Model file for the job. Use its own axes, mm. A direction names the side the tool comes from. Give positions to 0.01 mm unless a question says otherwise; leave off trailing zeros. Loops run counter-clockwise (first coordinate to the right, second up) from the corner with the lowest first, then second, coordinate; pieces in that order, holes last. Notation, with made-up numbers: M 5,12.5 L 29,12.5 A25 cw 29,30.5 Z; hole C -22.5,69 d5. An arc over 180 degrees is marked long. Answer in a Markdown table with one row per item.
```python
from build123d import *

# Parameters (mm, degrees)
ESBO_O1_W                = 20
ESBO_O1_H                = 25
RESSALTO_EXTRUS_O1_DEPTH = 9
ESBO_O2_R                = 7.5
CORTE_EXTRUS_O1_DEPTH    = 29.390139133
FILETE1_R                = 3
RESSALTO_EXTRUS_O2_DEPTH = 6
RESSALTO_EXTRUS_O3_DEPTH = 6
FILETE3_R                = 1
FILETE5_R                = 3
FILETE6_R                = 1
ESBO_O5_W                = 4
ESBO_O5_H                = 6
RESSALTO_EXTRUS_O4_DEPTH = 8


with BuildPart() as part:
    # Esboço1 → Ressalto-extrusão1 (new body)
    with BuildSketch(Plane(origin=(0, 0, 0), x_dir=(1, 0, 0), z_dir=(0, 1, 0))):
        Rectangle(ESBO_O1_W, ESBO_O1_H)
    extrude(amount=RESSALTO_EXTRUS_O1_DEPTH)

    # Esboço2 → Corte-extrusão1 (cut, through all)
    with BuildSketch(Plane.XY.offset(12.5)):
        with Locations((0, 10)):
            Circle(ESBO_O2_R)
    extrude(amount=-CORTE_EXTRUS_O1_DEPTH, mode=Mode.SUBTRACT)

    # Filete1
    filete1_edges = [part.edges().sort_by_distance(p)[0] for p in [
        (-10, 0, 0),
        (10, 0, 0),
    ]]
    fillet(filete1_edges, radius=FILETE1_R)

    # Esboço3 → Ressalto-extrusão2 (add)
    with BuildSketch(Plane(origin=(0, 9, 0), x_dir=(1, 0, 0), z_dir=(0, 1, 0))):
        Polygon((-16, 10), (-10, 10), (-10, 8.5), (-14, 8.5), (-14, 6.5), (-10, 6.5), (-10, 5), (-16, 5), align=None)
        Polygon((-14, -6.5), (-10, -6.5), (-10, -5), (-16, -5), (-16, -10), (-10, -10), (-10, -8.5), (-14, -8.5), align=None)
    extrude(amount=-RESSALTO_EXTRUS_O2_DEPTH)

    # Esboço4 → Ressalto-extrusão3 (add)
    with BuildSketch(Plane(origin=(0, 9, 0), x_dir=(1, 0, 0), z_dir=(0, 1, 0))):
        Polygon((-16, -10), (-16, -5), (-11, -5), (-11, -6.5), (-14, -6.5), (-14, -8.5), (-11, -8.5), (-11, -10), align=None)
        Polygon((-11, 10), (-16, 10), (-16, 5), (-11, 5), (-11, 6.5), (-14, 6.5), (-14, 8.5), (-11, 8.5), align=None)
    extrude(amount=RESSALTO_EXTRUS_O3_DEPTH)

    # Filete3
    filete3_edges = [part.edges().sort_by_distance(p)[0] for p in [
        (-16, 9, -5),
        (-16, 9, -10),
        (-16, 9, 10),
        (-16, 9, 5),
    ]]
    fillet(filete3_edges, radius=FILETE3_R)

    # Filete5
    # the kernel refuses this fillet: 3 mm, written as the material it adds along each edge
    with BuildSketch(Plane(origin=(-10, 16.5, -5), x_dir=(-1, 0, 0), z_dir=(0, -1, 0))) as filete5_piece_1_section:
        with BuildLine():
            CenterArc((FILETE5_R, -FILETE5_R), FILETE5_R, 90, 90)
            Line((0, -FILETE5_R), (0, 0))
            Line((0, 0), (FILETE5_R, 0))
        make_face()
    filete5_piece_1 = extrude(amount=13.5, mode=Mode.PRIVATE)
    filete5_piece_1 = split(filete5_piece_1, bisect_by=Plane(origin=(-11.589070595, 9, -4.827479681), z_dir=(0, 1, 0)), keep=Keep.TOP, mode=Mode.PRIVATE)
    filete5_piece_1 = split(filete5_piece_1, bisect_by=Plane(origin=(-11, 12, -4.827479681), z_dir=(-1, 0, 0)), keep=Keep.TOP, mode=Mode.PRIVATE)
    filete5_piece_1 = split(filete5_piece_1, bisect_by=Plane(origin=(-11.589070595, 15, -4.827479681), z_dir=(0, -1, 0)), keep=Keep.TOP, mode=Mode.PRIVATE)
    add(filete5_piece_1)
    with BuildSketch(Plane(origin=(-10, 9, -5), x_dir=(-1, 0, 0), z_dir=(0, -1, 0))) as filete5_piece_2_section:
        with BuildLine():
            CenterArc((FILETE5_R, -FILETE5_R), FILETE5_R, 90, 90)
            Line((0, -FILETE5_R), (0, 0))
            Line((0, 0), (FILETE5_R, 0))
        make_face()
    filete5_piece_2 = extrude(amount=6, mode=Mode.PRIVATE)
    filete5_piece_2 = split(filete5_piece_2, bisect_by=Plane(origin=(-11, 6, -4.827479681), z_dir=(-1, 0, 0)), keep=Keep.TOP, mode=Mode.PRIVATE)
    add(filete5_piece_2)
    with BuildSketch(Plane(origin=(-10, 9, -5), x_dir=(-1, 0, 0), z_dir=(0, -1, 0))) as filete5_piece_3_section:
        with BuildLine():
            CenterArc((FILETE5_R, -FILETE5_R), FILETE5_R, 90, 90)
            Line((0, -FILETE5_R), (0, 0))
            Line((0, 0), (FILETE5_R, 0))
        make_face()
    filete5_piece_3 = extrude(amount=6, mode=Mode.PRIVATE)
    filete5_piece_3 = split(filete5_piece_3, bisect_by=Plane(origin=(-11, 6, -4.141402177), z_dir=(1, 0, 0)), keep=Keep.TOP, mode=Mode.PRIVATE)
    add(filete5_piece_3)
    with BuildSketch(Plane(origin=(-10, 16.5, 5), x_dir=(-1, 0, 0), z_dir=(0, -1, 0))) as filete5_piece_4_section:
        with BuildLine():
            CenterArc((FILETE5_R, FILETE5_R), FILETE5_R, 180, 90)
            Line((0, FILETE5_R), (0, 0))
            Line((0, 0), (FILETE5_R, 0))
        make_face()
    filete5_piece_4 = extrude(amount=13.5, mode=Mode.PRIVATE)
    filete5_piece_4 = split(filete5_piece_4, bisect_by=Plane(origin=(-11.589070595, 15, 4.827479681), z_dir=(0, -1, 0)), keep=Keep.TOP, mode=Mode.PRIVATE)
    filete5_piece_4 = split(filete5_piece_4, bisect_by=Plane(origin=(-11.589070595, 9, 4.827479681), z_dir=(0, 1, 0)), keep=Keep.TOP, mode=Mode.PRIVATE)
    filete5_piece_4 = split(filete5_piece_4, bisect_by=Plane(origin=(-11, 12, 4.827479681), z_dir=(-1, 0, 0)), keep=Keep.TOP, mode=Mode.PRIVATE)
    add(filete5_piece_4)
    with BuildSketch(Plane(origin=(-10, 9, 5), x_dir=(-1, 0, 0), z_dir=(0, -1, 0))) as filete5_piece_5_section:
        with BuildLine():
            CenterArc((FILETE5_R, FILETE5_R), FILETE5_R, 180, 90)
            Line((0, FILETE5_R), (0, 0))
            Line((0, 0), (FILETE5_R, 0))
        make_face()
    filete5_piece_5 = extrude(amount=6, mode=Mode.PRIVATE)
    filete5_piece_5 = split(filete5_piece_5, bisect_by=Plane(origin=(-11, 6, 4.827479681), z_dir=(-1, 0, 0)), keep=Keep.TOP, mode=Mode.PRIVATE)
    add(filete5_piece_5)
    with BuildSketch(Plane(origin=(-10, 9, 5), x_dir=(-1, 0, 0), z_dir=(0, -1, 0))) as filete5_piece_6_section:
        with BuildLine():
            CenterArc((FILETE5_R, FILETE5_R), FILETE5_R, 180, 90)
            Line((0, FILETE5_R), (0, 0))
            Line((0, 0), (FILETE5_R, 0))
        make_face()
    filete5_piece_6 = extrude(amount=6, mode=Mode.PRIVATE)
    filete5_piece_6 = split(filete5_piece_6, bisect_by=Plane(origin=(-11, 6, 4.141402177), z_dir=(1, 0, 0)), keep=Keep.TOP, mode=Mode.PRIVATE)
    add(filete5_piece_6)

    # Filete6
    filete6_edges = [part.edges().sort_by_distance(p)[0] for p in [
        (-11, 12, -4.236067977),
        (-11, 12, 4.236067977),
    ]]
    fillet(filete6_edges, radius=FILETE6_R)

    # Esboço5 → Ressalto-extrusão4 (add)
    with BuildSketch(Plane(origin=(10, 0, 0), x_dir=(0, 0, -1), z_dir=(1, 0, 0))):
        with Locations((-10.5, 6)):
            Rectangle(ESBO_O5_W, ESBO_O5_H)
    extrude(amount=RESSALTO_EXTRUS_O4_DEPTH)


solid = part.part
```
Q1. Saw through at B-B (z = -7.5). Give the cut face in (x, y).
Reported:
| item | result |
|---|---|
| outline | M -16,3 L -14,3 L -14,15 L -16,15 Z; M -10,3 A3 ccw -7,0 L 7,0 A3 ccw 10,3 L 10,9 L 7.43,9 A7.5 cw -7.43,9 L -10,9 Z |
Q2. Saw through at A-A (y = 4.25). Give the number of separate pieces and of enclosed holes in the cut face, and give its area (3 significant figures).
Reported:
| item | result |
|---|---|
| separate pieces | 2 |
| enclosed holes | 2 |
| area | 338 mm² |
Q3. Drop flat-ended pins along their axis: pin 1 (2 mm diameter, centred on y = 6, z = 2, fed in from -X); pin 2 (1.6 mm diameter, centred on y = 11.5, z = 9, fed in from +X); pin 3 (8 mm diameter, centred on y = 5.5, z = -2.5, fed in from +X); pin 4 (8.5 mm diameter, centred on x = 15, z = 0, fed in from +Y). Give the stop position or say it passes through.
Reported:
| item | result |
|---|---|
| pin 1 | x = -10.17 |
| pin 2 | x = -11 |
| pin 3 | x = 10 |
| pin 4 | through |
Q4. Probe probe 1 along Z at (x, y) = (-13.5, 3.75); probe 2 along Z at (x, y) = (-11, 7.5); probe 3 along X at (y, z) = (11.75, -7.25). List the from-to ranges inside material, lowest first.
Reported:
| item | result |
|---|---|
| probe 1 | -10 to -8.5, -6.5 to -5, 5 to 6.5, 8.5 to 10 |
| probe 2 | -10 to -8.5, -6.5 to -4.24, 4.24 to 6.5, 8.5 to 10 |
| probe 3 | -16 to -14 |
Q5. 3-axis set-ups, long thin cutter, end or side, ignore diameter. For faces 1 (the face through (-13, 3, -6)), 2 (the face through (18, 6, 11)), 3 (the face through (-14, 9, 5)), 4 (the face through (-11, 12, 9)), 5 (the face through (-12, 9, -8.5)): which of +Z, -Z, +X, -X, +Y, -Y reach the whole face in a straight line?
Reported:
| item | result |
|---|---|
| face 1 | +Z, -Z, -X, -Y |
| face 2 | +Z, -Z, +X, +Y, -Y |
| face 3 | -X, +Y, -Y |
| face 4 | +Z, -Z, +X, +Y |
| face 5 | +Y, -Y |
Q6. Mould opens along Z. For faces 6 (the face through (14, 6, 8.5)), 7 (the face through (-10, 6, 0)), 8 (the face through (4, 3, 12.5)) say: released by +Z, released by -Z, zero draft, split by the parting line, or undercut.
Reported:
| item | result |
|---|---|
| face 6 | released by -Z |
| face 7 | undercut |
| face 8 | released by +Z |
Q7. Saw through at D-D (z = 11). Give the cut face in (x, y), and give its area (3 significant figures).
Reported:
| item | result |
|---|---|
| outline | M -10,3 A3 ccw -7,0 L 7,0 A3 ccw 10,3 L 18,3 L 18,9 L 7.43,9 A7.5 cw -7.43,9 L -10,9 Z |
| area | 151 mm² |
Q8. Saw through at C-C (y = 14.25). Give the cut face in (x, z), and give its area (3 significant figures).
Reported:
| item | result |
|---|---|
| outline | M -16,-9 A1 ccw -15,-10 L -11,-10 L -11,-8.5 L -14,-8.5 L -14,-6.5 L -11,-6.5 L -11,-5.87 A1 ccw -12.25,-4.9 A3 cw -13,-5 L -15,-5 A1 ccw -16,-6 Z; M -16,6 A1 ccw -15,5 L -13,5 A3 cw -12.25,4.9 A1 ccw -11,5.87 L -11,6.5 L -14,6.5 L -14,8.5 L -11,8.5 L -11,10 L -15,10 A1 ccw -16,9 Z |
| area | 37.1 mm² |
